```python
from build123d import *

# Parameters (mm, degrees)
SKETCH065_R  = 1
PAD047_DEPTH = 3
SKETCH056_R  = 3
PAD039_DEPTH = 10
SKETCH055_R  = 1.5
PAD038_DEPTH = 100
SKETCH057_R  = 1.5
PAD040_DEPTH = 100
SKETCH053_W  = 15.25
SKETCH053_H  = 6.793113
SKETCH054_W  = 8.25
SKETCH054_H  = 12.85529


with BuildPart() as pad047:
    # Sketch065 → Pad047 (new body)
    with BuildSketch(Plane.YZ.offset(31.5)):
        with Locations((2.75, -11)):
            Circle(SKETCH065_R)
        with Locations((-2.75, -11)):
            Circle(SKETCH065_R)
    extrude(amount=-PAD047_DEPTH)


with BuildPart() as mountingblockscrewcountersink:
    # Sketch056 → Pad039 (new body)
    with BuildSketch(Plane.XY.offset(-17)):
        with Locations((22, 4)):
            Circle(SKETCH056_R)
        with Locations((22, -4)):
            Circle(SKETCH056_R)
    extrude(amount=-PAD039_DEPTH)


with BuildPart() as mountingblockscrewcutout:
    # Sketch055 → Pad038 (new body)
    with BuildSketch(Plane.XY):
        with Locations((22, 4)):
            Circle(SKETCH055_R)
        with Locations((22, -4)):
            Circle(SKETCH055_R)
    extrude(amount=-PAD038_DEPTH)


with BuildPart() as cutouts:
    # Sketch057 → Pad040 (new body)
    with BuildSketch(Plane.XY):
        with Locations((28.75, 0)):
            Circle(SKETCH057_R)
        with Locations((18.75, 0)):
            Circle(SKETCH057_R)
    extrude(amount=-PAD040_DEPTH)

    # Fusion004011: union MountingBlockScrewCountersink, MountingBlockScrewCutout
    add(mountingblockscrewcountersink.part)
    add(mountingblockscrewcutout.part)


with BuildPart() as mountingblockpad:
    # Sketch053 → Loft003 section 0
    with BuildSketch(Plane.YZ.offset(16.5)):
        with Locations((0, -16.603444)):
            Rectangle(SKETCH053_W, SKETCH053_H)
    # Sketch054 → Loft003 section 1
    with BuildSketch(Plane.YZ.offset(31.5)):
        with Locations((0, -13.572355)):
            Rectangle(SKETCH054_W, SKETCH054_H)
    loft(ruled=True)

    # Cut007011: cut Cutouts
    add(cutouts.part, mode=Mode.SUBTRACT)

    # Cut007016: cut Pad047
    add(pad047.part, mode=Mode.SUBTRACT)


solid = mountingblockpad.part
```
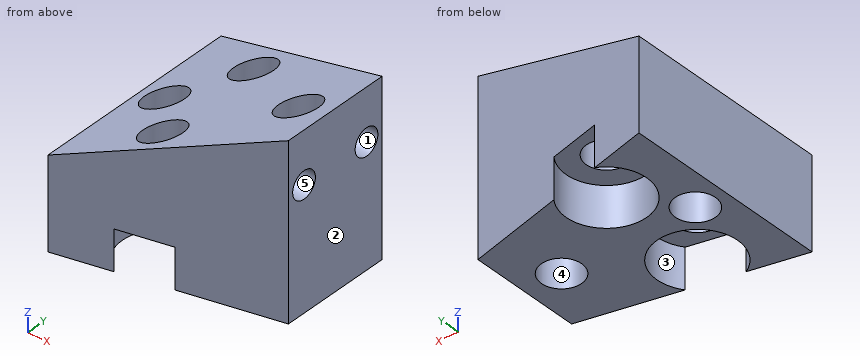
The model under review builds one solid part; all positions refer to its coordinate system, in mm. Face numbers are marked on the shaded views. A direction names the side the tool comes from. Round coordinates to 2 decimals unless told otherwise and drop trailing zeros. Write each question's results on one line, items separated by ' | '. Start each with the question number.
Q1. Insertion check: P1, Ø1, axis at x = 25.5, z = -18, coming from the -Y side; P2, Ø2.5, axis at y = -2.75, z = -11, coming from the -X side; P3, Ø2.5, axis at x = 22, y = 4, coming from the -Z side; P4, Ø5.5, axis at x = 22, y = 4, coming from the -Z side. Each pin has a flat end and moves straight along its axis. Give the tip position at first contact, or say it passes through.
Q2. Take a section at A-A on x = 29. Give the number of separate pieces and of enclosed holes in the cut face, plus the area to 3 significant figures.
Q3. Tool access review of the marked faces 3, 4 and 5: name each direction out of +Z, -Z, +X, -X, +Y, -Y from which nothing blocks a thin tool from reaching the whole face with its end or side.
Q4. Draft analysis for pull direction Y (two halves, no side actions). For the marked faces 1 and 2, state which applies: pulls with the +Y half, pulls with the -Y half, needs draft (parallel to the pull), parting line crosses it, or undercut.
Q5. Wall thickness on line 1 along Y through (x, z) = (22, -12.75); line 2 along X through (y, z) = (-0.5, -13.75); line 3 along Y through (x, z) = (22, -17.9): over which ranges is each line inside the solid? List them lowest first. Write a range as [from, to].
Data:
1) P1: stops at y = -5.64 | P2: stops at x = 18.87 | P3: passes through | P4: stops at z = -17
2) separate pieces: 2 | enclosed holes: 2 | area: 70.2 mm²
3) face 3: -Z | face 4: +Z, -Z | face 5: +X
4) face 1: undercut | face 2: needs draft
5) line 1: y = [-6.34, -5.5], [-2.5, 2.5], [5.5, 6.34] | line 2: x = [16.5, 17.34], [20.16, 27.34], [30.16, 31.5] | line 3: y = [-1, 1]
